For this review, take the finished solid that the model builds, in its own axes (mm). A direction names the side the tool comes from. Coordinates: 2 decimals unless noted, no trailing zeros. Order: outer loops, then holes, each group sorted by start corner. A loop starts at its lowest first (then second) coordinate and runs counter-clockwise, first axis right, second up. Notation, with made-up numbers: M 33.25,-6 L 50.25,-6 A16 ccw 50.25,24 Z; hole C 30,-12 d4. An arc over 180 degrees is marked long. Use CSV: the item, a comma, the result in double quotes.
```python
from build123d import *

# Parameters (mm, degrees)
SKETCH_1_W      = 110
SKETCH_1_H      = 32.5
SKETCH_2_R      = 4.325
EXTRUDE_1_DEPTH = 20
FILLET_1_R      = 2


with BuildPart() as part:
    # 스케치1 → 회전1 (revolve)
    with BuildSketch(Plane(origin=(0, 0, 0), x_dir=(1, 0, 0), z_dir=(0, 1, 0))):
        with Locations((0, 16.25)):
            Rectangle(SKETCH_1_W, SKETCH_1_H)
    revolve(axis=Axis((-130.174262735, 0, 0), (1, 0, 0)))

    # 스케치2 → 보스-돌출1 (add)
    with BuildSketch(Plane(origin=(55, 0, 0), x_dir=(0, 0, -1), z_dir=(1, 0, 0))):
        Circle(SKETCH_2_R)
    extrude_1 = extrude(amount=EXTRUDE_1_DEPTH)

    # 대칭 복사1: 보스-돌출1 across plane
    add(extrude_1.mirror(Plane(origin=(0, 0, 0), x_dir=(0, 0, 1), z_dir=(1, 0, 0))))

    # 필렛1
    fillet_1_edges = [part.edges().sort_by_distance(p)[0] for p in [
        (-55, 0, 4.325),
        (55, 0, 4.325),
    ]]
    fillet(fillet_1_edges, radius=FILLET_1_R)


solid = part.part
```
Item 1: Clearance check with flat-ended pins moving along their axes: pin 1 Ø4 at (x, y) = (-37, -24.5) entering from -Z; pin 2 Ø12 at (y, z) = (-19, -5) entering from -X; pin 3 Ø2 at (x, y) = (56.5, 2) entering from -Z. State where each tip first meets the part, or that it passes through.
Solutions:
pin 1,"z = -23.45"
pin 2,"x = -55"
pin 3,"z = -4.65"
Item 2: For faces 1 (the face through (65.874, 1.299, -4.125)), 2 (the face through (75, 0, 0)), list the 3-axis set-ups (+Z, -Z, +X, -X, +Y, -Y) from which the entire face can be reached by the end or side of a thin tool; tool diameter is ignored.
Solutions:
face 1,"+X"
face 2,"+Z, -Z, +X, +Y, -Y"
Item 3: To check wall thickness, follow line 1 along X through (y, z) = (-7, -23); line 2 along Z through (x, y) = (-1, -1); line 3 along Z through (x, y) = (-58, -2). State the ranges of each line that lie inside material, in increasing order. Write a range as [from, to].
Solutions:
line 1,"[-55, 55]"
line 2,"[-32.48, 32.48]"
line 3,"[-3.83, 3.83]"
Item 4: Add section C-C on x = 6.5. State the section outline as (y, z) points.
Solutions:
outline,"C 0,0 d65"
Item 5: Add section A-A on z = 0. State the section outline as (x, y) points (3 decimals).
Solutions:
outline,"M -75,-4.325 L -57,-4.325 A2 cw -55,-6.325 L -55,-32.5 L 55,-32.5 L 55,-6.325 A2 cw 57,-4.325 L 75,-4.325 L 75,4.325 L 57,4.325 A2 cw 55,6.325 L 55,32.5 L -55,32.5 L -55,6.325 A2 cw -57,4.325 L -75,4.325 Z"
Item 6: Draft analysis for pull direction X (two halves, no side actions). For faces 3 (the face through (55, 0, 7)), 4 (the face through (-65.874, 1.299, -4.125)), 5 (the face through (-55, 0, 7)), state which applies: released by +X, released by -X, zero draft, split by the parting line, or undercut.
Solutions:
face 3,"released by +X"
face 4,"zero draft"
face 5,"released by -X"
Item 7: Add section D-D on y = -26. State the section outline as (x, z) points.
Solutions:
outline,"M -55,-19.5 L 55,-19.5 L 55,19.5 L -55,19.5 Z"
